The listing builds one solid part. Answer for the finished solid, in the listing's coordinates (mm). Face numbers are marked on the shaded views. A direction names the side the tool comes from. Coordinates: 2 decimals unless noted, no trailing zeros. Order: outer loops, then holes, each group sorted by start corner. A loop starts at its lowest first (then second) coordinate and runs counter-clockwise, first axis right, second up. Notation, with made-up numbers: M 89,5 L 127,5 A29 cw 127,28 Z; hole C 40.5,1 d10. An arc over 180 degrees is marked long. One line per item, written item: value. Start each with the question number.
Q1. For the marked faces 1 and 2, determine the directions among +Z, -Z, +X, -X, +Y, -Y from which every point of the face is accessible in a straight line to the end or side of a thin tool.
Q2. The part is cut by section B-B on y = 8. Give the vertices of the cut face in (x, z).
Q3. Determine the mould class of the marked faces 3, 4 and 5 for opening direction Y: pulls with the +Y half, pulls with the -Y half, needs draft (parallel to the pull), parting line crosses it, or undercut.
Q4. The part is cut by section A-A on z = 0. Give the vertices of the cut face in (x, y).
Q5. The part is cut by section C-C on z = -9. Give the vertices of the cut face in (x, y).
Q6. The part is cut by section D-D on x = 9. Give the vertices of the cut face in (y, z), then the cut area to 3 significant figures.
Q7. Straight lines are drawn through the part: line 1 along Y through (x, z) = (0.95, 0); line 2 along X through (y, z) = (4.5, -6); line 3 along Y through (x, z) = (9.5, -1.25). For each, find the intervals that lie inside material, in ascending order. Write a range as [from, to].
Q8. Each of these flat-tipped pins is pushed along its axis until it touches: pin 1 Ø6 at (x, y) = (9, 5.5) entering from -Z; pin 2 Ø5 at (y, z) = (-8, -0.002) entering from +X. Where does it stop, or does it pass through?
```python
from build123d import *

# Parameters (mm, degrees)
SKETCH_1_R          = 11
EXTRUDE_1_DEPTH     = 2
SKETCH_2_R          = 5
SKETCH_2_R_2        = 2.5
EXTRUDE_2_DEPTH     = 10
SKETCH_3_R          = 1.5
CUT_EXTRUDE_1_DEPTH = 10
SKETCH_5_R          = 2.5
CUT_EXTRUDE_2_DEPTH = 19.493242009


with BuildPart() as part:
    # 草图1 → 凸台-拉伸1 (new body)
    with BuildSketch(Plane(origin=(0, 0, 0), x_dir=(0, 0, -1), z_dir=(1, 0, 0))):
        Circle(SKETCH_1_R)
    extrude(amount=EXTRUDE_1_DEPTH)

    # 草图2 → 凸台-拉伸2 (add)
    with BuildSketch(Plane(origin=(2, 0, 0), x_dir=(0, 0, -1), z_dir=(1, 0, 0))):
        Circle(SKETCH_2_R)
        Circle(SKETCH_2_R_2, mode=Mode.SUBTRACT)
    extrude(amount=EXTRUDE_2_DEPTH)

    # 草图3 → 切除-拉伸1 (cut)
    with BuildSketch(Plane(origin=(2, 0, 0), x_dir=(0, 0, -1), z_dir=(1, 0, 0))):
        with Locations((0, 8)):
            Circle(SKETCH_3_R)
        with Locations((8.001, 0.001)):
            Circle(SKETCH_3_R)
        with Locations((0.002, -8)):
            Circle(SKETCH_3_R)
        with Locations((-7.999, -0.001)):
            Circle(SKETCH_3_R)
    extrude(amount=-CUT_EXTRUDE_1_DEPTH, mode=Mode.SUBTRACT)

    # 草图5 → 切除-拉伸2 (cut, through all)
    with BuildSketch(Plane(origin=(2, 0, 0), x_dir=(0, 0, -1), z_dir=(1, 0, 0))):
        Circle(SKETCH_5_R)
    extrude(amount=-CUT_EXTRUDE_2_DEPTH, mode=Mode.SUBTRACT)


solid = part.part
```
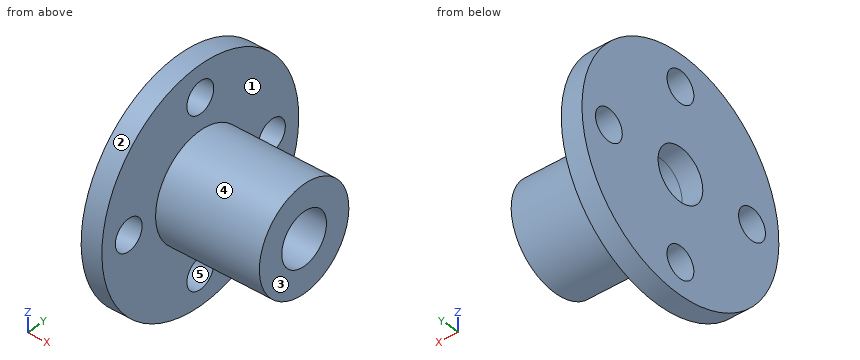
Output:
1. face 1: +X
1. face 2: +X, -X
2. outline: M 0,-7.55 L 2,-7.55 L 2,-1.5 L 0,-1.5 Z; M 0,1.5 L 2,1.5 L 2,7.55 L 0,7.55 Z
3. face 3: needs draft
3. face 4: parting line crosses it
3. face 5: undercut
4. outline: M 0,-11 L 2,-11 L 2,-9.5 L 0,-9.5 Z; M 0,-6.5 L 2,-6.5 L 2,-5 L 12,-5 L 12,-2.5 L 0,-2.5 Z; M 0,2.5 L 12,2.5 L 12,5 L 2,5 L 2,6.5 L 0,6.5 Z; M 0,9.5 L 2,9.5 L 2,11 L 0,11 Z
5. outline: M 0,-6.32 L 2,-6.32 L 2,-1.12 L 0,-1.12 Z; M 0,1.12 L 2,1.12 L 2,6.32 L 0,6.32 Z
6. outline: C 0,0 d10; hole C 0,0 d5
6. area: 58.9 mm^2
7. line 1: y = [-11, -9.5], [-6.5, -2.5], [2.5, 6.5], [9.5, 11]
7. line 2: x = [0, 2]
7. line 3: y = [-4.84, -2.17], [2.17, 4.84]
8. pin 1: stops at z = -4.33
8. pin 2: stops at x = 2
